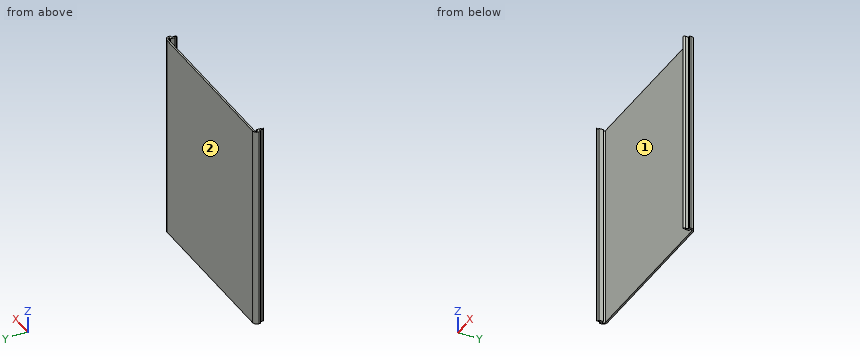
from build123d import *

# Parameters (mm, degrees)
MAINBODY_DEPTH = 304.8


with BuildPart() as part:
    # Sketch2 → MainBody (new body)
    with BuildSketch(Plane.XY):
        with BuildLine():
            Line((-119.888, -15.748740175), (-119.881210728, -14.923222028))
            ThreePointArc((-119.881210728, -14.923222028), (-121.097875098, -13.267102575), (-119.146762684, -12.621994695))
            Line((-119.146762684, -12.621994695), (-118.992266474, -12.621994695))
            Line((-118.992266474, -12.621994695), (-118.992266474, -6.004220787))
            Line((-118.992266474, -6.004220787), (-122.428, -6.004220787))
            Line((-122.428, -6.004220787), (-122.428, -5.715))
            ThreePointArc((-122.428, -5.715), (-121.49806403, -3.46993597), (-119.253, -2.54))
            Line((-119.253, -2.54), (119.253, -2.54))
            ThreePointArc((119.253, -2.54), (121.49806403, -3.46993597), (122.428, -5.715))
            Line((122.428, -5.715), (122.428, -6.004220787))
            Line((122.428, -6.004220787), (118.992266474, -6.004220787))
            Line((118.992266474, -6.004220787), (118.992266474, -12.621994695))
            Line((118.992266474, -12.621994695), (119.146762684, -12.621994695))
            ThreePointArc((119.146762684, -12.621994695), (121.097875098, -13.267102575), (119.881210728, -14.923222028))
            Line((119.881210728, -14.923222028), (119.888, -15.748740175))
            ThreePointArc((119.888, -15.748740175), (121.651583177, -14.78500633), (121.793, -12.780259505))
            Line((121.793, -12.780259505), (121.793, -8.665459505))
            Line((121.793, -8.665459505), (124.968, -8.665459505))
            Line((124.968, -8.665459505), (124.968, -6.35))
            ThreePointArc((124.968, -6.35), (123.108128061, -1.859871939), (118.618, 0))
            Line((118.618, 0), (-118.618, 0))
            ThreePointArc((-118.618, 0), (-123.108128061, -1.859871939), (-124.968, -6.35))
            Line((-124.968, -6.35), (-124.968, -8.665459505))
            Line((-124.968, -8.665459505), (-121.793, -8.665459505))
            Line((-121.793, -8.665459505), (-121.793, -12.780259505))
            ThreePointArc((-121.793, -12.780259505), (-121.651583177, -14.78500633), (-119.888, -15.748740175))
        make_face()
    extrude(amount=MAINBODY_DEPTH)


solid = part.part
Verification items for the finished model (mm, model axes). Face numbers are marked on the shaded views. Round coordinates to 2 decimals unless told otherwise and drop trailing zeros. Loops run counter-clockwise (first coordinate to the right, second up) from the corner with the lowest first, then second, coordinate; pieces in that order, holes last. Notation, with made-up numbers: (59, -22.75) - (106, -22.75) arc R16 cw to (106, -14.75) - close; hole circle Ø6 at (38.5, -6). An arc over 180 degrees is marked (long way). Use a Markdown table: item, result. Add a question column.
1. Release check for a two-part mould opening along X. For the marked faces 1 and 2 record: released by +X, released by -X, zero draft, split by the parting line, or undercut.
2. Gauge pin test, flat ends, axial feed: pin 1 (10 mm diameter, centred on x = 25, z = 227.5, fed in from -Y); pin 2 (2.5 mm diameter, centred on x = -123, z = 130, fed in from -Y); pin 3 (2 mm diameter, centred on y = -14, z = 38, fed in from +X). Record the tip position at first contact, or that the pin passes through.
3. Thickness scan on probe 1 along X at (y, z) = (-10.5, 191); probe 2 along X at (y, z) = (-13.25, 74); probe 3 along Y at (x, z) = (94, 143). Record the ranges inside material, lowest first. Write a range as [from, to].
4. Section check B-B, the plane x = 80. Record the boundary of the cut face in (y, z).
Checks:
| question | item | result |
|---|---|---|
| 1 | face 1 | undercut |
| 1 | face 2 | zero draft |
| 2 | pin 1 | stops at y = -2.54 |
| 2 | pin 2 | stops at y = -14.61 |
| 2 | pin 3 | stops at x = 121.98 |
| 3 | probe 1 | x = [-121.79, -118.99], [118.99, 121.79] |
| 3 | probe 2 | x = [-121.94, -121.09], [121.09, 121.94] |
| 3 | probe 3 | y = [-2.54, 0] |
| 4 | outline | (-2.54, 0) - (0, 0) - (0, 304.8) - (-2.54, 304.8) - close |
